from build123d import *

# Parameters (mm, degrees)
BOX007_W          = 63
BOX007_H          = 37
BOX007_DEPTH      = 5.5
BOX006_W          = 10
BOX006_H          = 8
BOX006_DEPTH      = 5.5
CYLINDER016_R     = 3.25
CYLINDER016_DEPTH = 3
CYLINDER017_R     = 1.5
CYLINDER017_DEPTH = 8.5
CYLINDER018_R     = 5.25
CYLINDER018_DEPTH = 8.5
CYLINDER014_R     = 3.25
CYLINDER014_DEPTH = 3
CYLINDER013_R     = 1.5
CYLINDER013_DEPTH = 8.5
CYLINDER015_R     = 5.25
CYLINDER015_DEPTH = 8.5
CYLINDER010_R     = 3.25
CYLINDER010_DEPTH = 3
CYLINDER009_R     = 1.5
CYLINDER009_DEPTH = 8.5
CYLINDER008_R     = 5.25
CYLINDER008_DEPTH = 8.5
CYLINDER021_R     = 3.25
CYLINDER021_DEPTH = 3
CYLINDER020_R     = 1.5
CYLINDER020_DEPTH = 8.5
CYLINDER019_R     = 5.25
CYLINDER019_DEPTH = 8.5
CYLINDER023_R     = 3.25
CYLINDER023_DEPTH = 3
CYLINDER022_R     = 1.5
CYLINDER022_DEPTH = 8.5
CYLINDER025_R     = 3.25
CYLINDER025_DEPTH = 3
CYLINDER024_R     = 1.5
CYLINDER024_DEPTH = 8.5
CYLINDER026_R     = 3.25
CYLINDER026_DEPTH = 3
CYLINDER027_R     = 1.5
CYLINDER027_DEPTH = 8.5
CYLINDER029_R     = 3.25
CYLINDER029_DEPTH = 3
CYLINDER028_R     = 1.5
CYLINDER028_DEPTH = 8.5
BOX_W             = 63
BOX_H             = 37
BOX_DEPTH         = 6
BOX001_W          = 10
BOX001_H          = 8
BOX001_DEPTH      = 6
BOX002_W          = 69
BOX002_H          = 43
BOX002_DEPTH      = 8.5


with BuildPart() as cube006:
    # Box007 → Box007 (new body)
    with BuildSketch(Plane.XY):
        with Locations((31.5, 18.5)):
            Rectangle(BOX007_W, BOX007_H)
    extrude(amount=BOX007_DEPTH)


with BuildPart() as battery_model002:
    # Box006 → Box006 (new body)
    with BuildSketch(Plane(origin=(63, 16, 0), x_dir=(1, 0, 0), z_dir=(0, 0, 1))):
        with Locations((5, 4)):
            Rectangle(BOX006_W, BOX006_H)
    extrude(amount=BOX006_DEPTH)

    # Fusion012: union Cube006
    add(cube006.part)


with BuildPart() as battery_model002_1:
    # Fusion012 placement: moved
    add(battery_model002.part.moved(Location((3, 3, 3))))


with BuildPart() as nut_recess002:
    # Cylinder016 → Cylinder016 (new body)
    with BuildSketch(Plane(origin=(15, -1, 0), x_dir=(1, 0, 0), z_dir=(0, 0, 1))):
        Circle(CYLINDER016_R)
    extrude(amount=CYLINDER016_DEPTH)


with BuildPart() as base_bolt_assembly002:
    # Cylinder017 → Cylinder017 (new body)
    with BuildSketch(Plane(origin=(15, -1, 0), x_dir=(1, 0, 0), z_dir=(0, 0, 1))):
        Circle(CYLINDER017_R)
    extrude(amount=CYLINDER017_DEPTH)

    # Fusion004: union Nut Recess002
    add(nut_recess002.part)


with BuildPart() as obj1:
    # Cylinder018 → Cylinder018 (new body)
    with BuildSketch(Plane(origin=(15, -1, 0), x_dir=(1, 0, 0), z_dir=(0, 0, 1))):
        Circle(CYLINDER018_R)
    extrude(amount=CYLINDER018_DEPTH)

    # Cut005: cut Base Bolt Assembly002
    add(base_bolt_assembly002.part, mode=Mode.SUBTRACT)


with BuildPart() as obj1_1:
    # Cut005 placement: moved
    add(obj1.part.moved(Location((39, 45, 0))))


with BuildPart() as nut_recess001:
    # Cylinder014 → Cylinder014 (new body)
    with BuildSketch(Plane(origin=(15, -1, 0), x_dir=(1, 0, 0), z_dir=(0, 0, 1))):
        Circle(CYLINDER014_R)
    extrude(amount=CYLINDER014_DEPTH)


with BuildPart() as base_bolt_assembly001:
    # Cylinder013 → Cylinder013 (new body)
    with BuildSketch(Plane(origin=(15, -1, 0), x_dir=(1, 0, 0), z_dir=(0, 0, 1))):
        Circle(CYLINDER013_R)
    extrude(amount=CYLINDER013_DEPTH)

    # Fusion003: union Nut Recess001
    add(nut_recess001.part)


with BuildPart() as obj2:
    # Cylinder015 → Cylinder015 (new body)
    with BuildSketch(Plane(origin=(15, -1, 0), x_dir=(1, 0, 0), z_dir=(0, 0, 1))):
        Circle(CYLINDER015_R)
    extrude(amount=CYLINDER015_DEPTH)

    # Cut004: cut Base Bolt Assembly001
    add(base_bolt_assembly001.part, mode=Mode.SUBTRACT)


with BuildPart() as obj2_1:
    # Cut004 placement: moved
    add(obj2.part.moved(Location((39, 0, 0))))


with BuildPart() as nut_recess:
    # Cylinder010 → Cylinder010 (new body)
    with BuildSketch(Plane(origin=(15, -1, 0), x_dir=(1, 0, 0), z_dir=(0, 0, 1))):
        Circle(CYLINDER010_R)
    extrude(amount=CYLINDER010_DEPTH)


with BuildPart() as base_bolt_assembly:
    # Cylinder009 → Cylinder009 (new body)
    with BuildSketch(Plane(origin=(15, -1, 0), x_dir=(1, 0, 0), z_dir=(0, 0, 1))):
        Circle(CYLINDER009_R)
    extrude(amount=CYLINDER009_DEPTH)

    # Fusion002: union Nut Recess
    add(nut_recess.part)


with BuildPart() as obj3:
    # Cylinder008 → Cylinder008 (new body)
    with BuildSketch(Plane(origin=(15, -1, 0), x_dir=(1, 0, 0), z_dir=(0, 0, 1))):
        Circle(CYLINDER008_R)
    extrude(amount=CYLINDER008_DEPTH)

    # Cut002: cut Base Bolt Assembly
    add(base_bolt_assembly.part, mode=Mode.SUBTRACT)


with BuildPart() as nut_recess003:
    # Cylinder021 → Cylinder021 (new body)
    with BuildSketch(Plane(origin=(15, -1, 0), x_dir=(1, 0, 0), z_dir=(0, 0, 1))):
        Circle(CYLINDER021_R)
    extrude(amount=CYLINDER021_DEPTH)


with BuildPart() as base_bolt_assembly003:
    # Cylinder020 → Cylinder020 (new body)
    with BuildSketch(Plane(origin=(15, -1, 0), x_dir=(1, 0, 0), z_dir=(0, 0, 1))):
        Circle(CYLINDER020_R)
    extrude(amount=CYLINDER020_DEPTH)

    # Fusion005: union Nut Recess003
    add(nut_recess003.part)


with BuildPart() as base_bolt_assemblies_no_bat:
    # Cylinder019 → Cylinder019 (new body)
    with BuildSketch(Plane(origin=(15, -1, 0), x_dir=(1, 0, 0), z_dir=(0, 0, 1))):
        Circle(CYLINDER019_R)
    extrude(amount=CYLINDER019_DEPTH)

    # Cut006: cut Base Bolt Assembly003
    add(base_bolt_assembly003.part, mode=Mode.SUBTRACT)


with BuildPart() as base_bolt_assemblies_no_bat_1:
    # Cut006 placement: moved
    add(base_bolt_assemblies_no_bat.part.moved(Location((0, 45, 0))))

    # Fusion011: union obj1, obj2, obj3
    add(obj1_1.part)
    add(obj2_1.part)
    add(obj3.part)

    # Cut008: cut Battery Model002
    add(battery_model002_1.part, mode=Mode.SUBTRACT)


with BuildPart() as nut_recess004:
    # Cylinder023 → Cylinder023 (new body)
    with BuildSketch(Plane(origin=(15, -1, 0), x_dir=(1, 0, 0), z_dir=(0, 0, 1))):
        Circle(CYLINDER023_R)
    extrude(amount=CYLINDER023_DEPTH)


with BuildPart() as obj4:
    # Cylinder022 → Cylinder022 (new body)
    with BuildSketch(Plane(origin=(15, -1, 0), x_dir=(1, 0, 0), z_dir=(0, 0, 1))):
        Circle(CYLINDER022_R)
    extrude(amount=CYLINDER022_DEPTH)

    # Fusion006: union Nut Recess004
    add(nut_recess004.part)


with BuildPart() as nut_recess005:
    # Cylinder025 → Cylinder025 (new body)
    with BuildSketch(Plane(origin=(15, -1, 0), x_dir=(1, 0, 0), z_dir=(0, 0, 1))):
        Circle(CYLINDER025_R)
    extrude(amount=CYLINDER025_DEPTH)


with BuildPart() as obj5:
    # Cylinder024 → Cylinder024 (new body)
    with BuildSketch(Plane(origin=(15, -1, 0), x_dir=(1, 0, 0), z_dir=(0, 0, 1))):
        Circle(CYLINDER024_R)
    extrude(amount=CYLINDER024_DEPTH)

    # Fusion007: union Nut Recess005
    add(nut_recess005.part)


with BuildPart() as obj5_1:
    # Fusion007 placement: moved
    add(obj5.part.moved(Location((39, 0, 0))))


with BuildPart() as nut_recess006:
    # Cylinder026 → Cylinder026 (new body)
    with BuildSketch(Plane(origin=(15, -1, 0), x_dir=(1, 0, 0), z_dir=(0, 0, 1))):
        Circle(CYLINDER026_R)
    extrude(amount=CYLINDER026_DEPTH)


with BuildPart() as obj6:
    # Cylinder027 → Cylinder027 (new body)
    with BuildSketch(Plane(origin=(15, -1, 0), x_dir=(1, 0, 0), z_dir=(0, 0, 1))):
        Circle(CYLINDER027_R)
    extrude(amount=CYLINDER027_DEPTH)

    # Fusion008: union Nut Recess006
    add(nut_recess006.part)


with BuildPart() as obj6_1:
    # Fusion008 placement: moved
    add(obj6.part.moved(Location((39, 45, 0))))


with BuildPart() as nut_recess007:
    # Cylinder029 → Cylinder029 (new body)
    with BuildSketch(Plane(origin=(15, -1, 0), x_dir=(1, 0, 0), z_dir=(0, 0, 1))):
        Circle(CYLINDER029_R)
    extrude(amount=CYLINDER029_DEPTH)


with BuildPart() as base_bolt_remove_assembly:
    # Cylinder028 → Cylinder028 (new body)
    with BuildSketch(Plane(origin=(15, -1, 0), x_dir=(1, 0, 0), z_dir=(0, 0, 1))):
        Circle(CYLINDER028_R)
    extrude(amount=CYLINDER028_DEPTH)

    # Fusion009: union Nut Recess007
    add(nut_recess007.part)


with BuildPart() as base_bolt_remove_assembly_1:
    # Fusion009 placement: moved
    add(base_bolt_remove_assembly.part.moved(Location((0, 45, 0))))

    # Fusion010: union obj4, obj5, obj6
    add(obj4.part)
    add(obj5_1.part)
    add(obj6_1.part)


with BuildPart() as cube:
    # Box → Box (new body)
    with BuildSketch(Plane.XY):
        with Locations((31.5, 18.5)):
            Rectangle(BOX_W, BOX_H)
    extrude(amount=BOX_DEPTH)


with BuildPart() as battery_model:
    # Box001 → Box001 (new body)
    with BuildSketch(Plane(origin=(63, 16, 0), x_dir=(1, 0, 0), z_dir=(0, 0, 1))):
        with Locations((5, 4)):
            Rectangle(BOX001_W, BOX001_H)
    extrude(amount=BOX001_DEPTH)

    # Fusion: union Cube
    add(cube.part)


with BuildPart() as battery_model_1:
    # Fusion placement: moved
    add(battery_model.part.moved(Location((3, 3, 3))))


with BuildPart() as base_initial:
    # Box002 → Box002 (new body)
    with BuildSketch(Plane.XY):
        with Locations((34.5, 21.5)):
            Rectangle(BOX002_W, BOX002_H)
    extrude(amount=BOX002_DEPTH)

    # Cut: cut Battery Model
    add(battery_model_1.part, mode=Mode.SUBTRACT)

    # Cut007: cut Base Bolt Remove Assembly
    add(base_bolt_remove_assembly_1.part, mode=Mode.SUBTRACT)

    # Fusion013: union Base Bolt Assemblies - no Bat
    add(base_bolt_assemblies_no_bat_1.part)


solid = base_initial.part
The listing builds one solid part. Answer for the finished solid, in the listing's coordinates (mm). A direction names the side the tool comes from. Coordinates: 2 decimals unless noted, no trailing zeros. Loops run counter-clockwise (first coordinate to the right, second up) from the corner with the lowest first, then second, coordinate; pieces in that order, holes last.
1) Find section B-B on z = 1. Write down the section's boundary in (x, y), then the cut area to 3 significant figures.
2) Flat-ended cylindrical pins translate along their axes: pin 1 Ø3 at (x, z) = (18, 4) entering from -Y; pin 2 Ø2.5 at (x, y) = (54, -1) entering from +Z; pin 3 Ø4 at (x, z) = (48, 5.5) entering from -Y; pin 4 Ø2.5 at (x, z) = (62, 6) entering from -Y. Find the tip coordinate at first contact, or state that the pin passes through.
3) Find section A-A on x = 54. Write down the section's boundary in (y, z), then the cut area to 3 significant figures.
4) Find section C-C on y = -1. Write down the section's boundary in (x, z).
5) Find the intervals of material crossed by L1, parallel to Y at x = 54, z = 0.85; L2, parallel to Y at x = 30, z = 6.25; L3, parallel to X at y = 44, z = 6.15, in increasing order.
6) A tool of negligible diameter and unlimited length cuts with its end or side. For faces 1 (the face through (66, 33, 6)), 2 (the face through (13.5, -0.93, 5.71)), 3 (the face through (50.753, -0.857, 1.479)), from which of +Z, -Z, +X, -X, +Y, -Y can it reach the whole face along a straight path? Write none if from no direction.
7) Find section D-D on x = 27.5. Write down the section's boundary in (y, z).
Values:
1. outline: (0, 0) - (9.85, 0) arc R5.25 ccw (long way) to (20.15, 0) - (48.85, 0) arc R5.25 ccw (long way) to (59.15, 0) - (69, 0) - (69, 43) - (59.15, 43) arc R5.25 ccw (long way) to (48.85, 43) - (20.15, 43) arc R5.25 ccw (long way) to (9.85, 43) - (0, 43) - close; hole circle Ø6.5 at (15, -1); hole circle Ø6.5 at (15, 44); hole circle Ø6.5 at (54, -1); hole circle Ø6.5 at (54, 44)
1. area: 3,050 mm2
2. pin 1: stops at y = -6.03
2. pin 2: passes through
2. pin 3: stops at y = -4.4
2. pin 4: stops at y = 0
3. outline: (-6.25, 0) - (-4.25, 0) - (-4.25, 3) - (-2.5, 3) - (-2.5, 8.5) - (-6.25, 8.5) - close; (0.5, 3) - (2.25, 3) - (2.25, 0) - (40.75, 0) - (40.75, 3) - (42.5, 3) - (42.5, 8.5) - (40, 8.5) - (40, 3) - (3, 3) - (3, 8.5) - (0.5, 8.5) - close; (45.5, 3) - (47.25, 3) - (47.25, 0) - (49.25, 0) - (49.25, 8.5) - (45.5, 8.5) - close
3. area: 196 mm2
4. outline: (9.75, 0) - (11.75, 0) - (11.75, 3) - (13.5, 3) - (13.5, 8.5) - (9.75, 8.5) - close; (16.5, 3) - (18.25, 3) - (18.25, 0) - (20.25, 0) - (20.25, 8.5) - (16.5, 8.5) - close; (48.75, 0) - (50.75, 0) - (50.75, 3) - (52.5, 3) - (52.5, 8.5) - (48.75, 8.5) - close; (55.5, 3) - (57.25, 3) - (57.25, 0) - (59.25, 0) - (59.25, 8.5) - (55.5, 8.5) - close
5. L1: y = -6.25 to -4.25, 2.25 to 40.75, 47.25 to 49.25
5. L2: y = 0 to 3, 40 to 43
5. L3: x = 9.75 to 13.5, 16.5 to 20.25, 48.75 to 52.5, 55.5 to 59.25
6. face 1: +Z
6. face 2: +Z, -Z
6. face 3: -Z
7. outline: (0, 0) - (43, 0) - (43, 8.5) - (40, 8.5) - (40, 3) - (3, 3) - (3, 8.5) - (0, 8.5) - close
